Verification items for the finished model (mm, model axes). A direction names the side the tool comes from. Round coordinates to 2 decimals unless told otherwise and drop trailing zeros. Order: outer loops, then holes, each group sorted by start corner. A loop starts at its lowest first (then second) coordinate and runs counter-clockwise, first axis right, second up. Notation, with made-up numbers: M 71,31.25 L 125,31.25 A15 cw 125,57.25 Z; hole C -27.5,-5 d7. An arc over 180 degrees is marked long. One line per item, written item: value. Start each with the question number.
from build123d import *

# Parameters (mm, degrees)
F0_W        = 152.4
F0_H        = 76.2
F1_DEPTH    = 12.7
F2_R        = 6.35
F3_DEPTH    = 12.701
F4_W        = 25.4
F4_H        = 50.8
F6_W        = 11.3594501876
F6_H        = 17.78
F8_R        = 5.08
F9_T1_DEPTH = 102.3282991577
F9_T3_DEPTH = 178.5282991577


# Not quite as in the source:
# - a fillet or chamfer that OpenCascade refuses, or shapes differently, is made with other operations: its cross-section is extruded or revolved along the edge and cut away or added


with BuildPart() as f1:
    # F0 (on Top) → F1 (new body)
    with BuildSketch(Plane.XY):
        Rectangle(F0_W, F0_H)
    extrude(amount=F1_DEPTH)

    # F2 (on face) → F3 (cut, through all)
    with BuildSketch(Plane.XY.offset(12.7)):
        with Locations((-63.9521719884, 28.7373781539)):
            Circle(F2_R)
        with Locations((-65.762154874, -27.1426218461)):
            Circle(F2_R)
        with Locations((63.0478280116, 28.7373781539)):
            Circle(F2_R)
        with Locations((61.237845126, -27.1426218461)):
            Circle(F2_R)
    extrude(amount=-F3_DEPTH, mode=Mode.SUBTRACT)

    # F4 (on Front) → F5 (revolve)
    with BuildSketch(Plane.XZ):
        with Locations((12.7, 38.1)):
            Rectangle(F4_W, F4_H)
    revolve(axis=Axis((0, 0, 38.1), (0, 0, 1)))

    # F6 (on Front) → F7 (revolve, cut)
    with BuildSketch(Plane.XZ):
        with Locations((25.2974471077, 38.0985615775)):
            Rectangle(F6_W, F6_H)
    revolve(axis=Axis((0, 0, 12.7), (0, 0, 1)), mode=Mode.SUBTRACT)

    # F8
    f8_edges = [f1.edges().sort_by_distance(p)[0] for p in [
        (-25.4, 0, 63.5),
        (-25.4, 0, 12.7),
    ]]
    fillet(f8_edges, radius=F8_R)

    # F9: chamfer of 5.08 on 4 edges, made by hand

    # F9_s2 → F9_t1 (cut)
    with BuildSketch(Plane.XZ.offset(-51.1641495789)):
        Polygon((71.12, 12.7), (76.2, 7.62), (76.2, 12.7), align=None)
        Polygon((-71.12, 12.7), (-76.2, 7.62), (-76.2, 12.7), align=None)
    extrude(amount=F9_T1_DEPTH, mode=Mode.SUBTRACT)

    # F9_s4 → F9_t3 (cut)
    with BuildSketch(Plane.YZ.offset(-89.2641495789)):
        Polygon((33.02, 12.7), (38.1, 7.62), (38.1, 12.7), align=None)
        Polygon((-33.02, 12.7), (-38.1, 7.62), (-38.1, 12.7), align=None)
    extrude(amount=F9_T3_DEPTH, mode=Mode.SUBTRACT)


solid = f1.part
1. Depth check by flat-ended pin: pin 1 (4 mm diameter, centred on y = -13, z = 55, fed in from +X); pin 2 (20.5 mm diameter, centred on x = -63.95, y = 28.74, fed in from +Z); pin 3 (5 mm diameter, centred on x = -19.5, z = 35, fed in from -Y); pin 4 (12 mm diameter, centred on x = -16, y = -1, fed in from -Z). Enter the tip coordinate at first touch or a pass-through.
2. Draft check along Y on faces 1 (the face through (73.62, 0.53, 10.2)), 2 (the face through (-65.33, 22.54, 6.44)), 3 (the face through (-1.07, 35.52, 10.2)), 4 (the face through (-59.896, -29.575, 6.439)). Enter one of: released by +Y, released by -Y, zero draft, split by the parting line, or undercut.
3. Section check C-C (z = 35). Record the cut outline in (x, y).
4. Scan lines: line 1 along X through (y, z) = (25.5, 4); line 2 along X through (y, z) = (-29.5, 5.5); line 3 along Z through (x, y) = (-36.5, -24.5). Record each from-to range of solid material in increasing order.
5. Section check A-A (x = 0). Record the cut outline in (y, z), and give its area (3 significant figures).
6. Tool access check on faces 5 (the face through (-1.07, -35.52, 10.2)), 6 (the face through (-13, -15, 29.209)), 7 (the face through (-5.506, -24.796, 23.574)). Record the directions out of +Z, -Z, +X, -X, +Y, -Y that give a thin tool (end or side, any length) a straight path to the whole face; none if there is none.
7. Section check B-B (z = 6). Record the cut outline in (x, y), and give its area (3 significant figures).
8. Section check D-D (z = 53). Record the cut outline in (x, y), and give its area (3 significant figures).
Geometry check:
1. pin 1: stops at x = 22.89
1. pin 2: stops at z = 12.7
1. pin 3: stops at y = -9.79
1. pin 4: stops at z = 0
2. face 1: zero draft
2. face 2: undercut
2. face 3: released by +Y
2. face 4: undercut
3. outline: C 0,0 d39.24
4. line 1: x = -76.2 to -69.41, -58.49 to 57.59, 68.51 to 76.2
4. line 2: x = -76.2 to -71.66, -59.87 to 55.34, 67.13 to 76.2
4. line 3: z = 0 to 12.7
5. outline: M -38.1,0 L 38.1,0 L 38.1,7.62 L 33.02,12.7 L 30.48,12.7 A5.08 cw 25.4,17.78 L 25.4,29.21 L 19.62,29.21 L 19.62,46.99 L 25.4,46.99 L 25.4,58.42 A5.08 ccw 20.32,63.5 L -20.32,63.5 A5.08 ccw -25.4,58.42 L -25.4,46.99 L -19.62,46.99 L -19.62,29.21 L -25.4,29.21 L -25.4,17.78 A5.08 cw -30.48,12.7 L -33.02,12.7 L -38.1,7.62 Z
5. area: 3,320 mm²
6. face 5: +Z, +X, -X, -Y
6. face 6: none
6. face 7: +Z
7. outline: M -76.2,-38.1 L 76.2,-38.1 L 76.2,38.1 L -76.2,38.1 Z; hole C -65.76,-27.14 d12.7; hole C -63.95,28.74 d12.7; hole C 61.24,-27.14 d12.7; hole C 63.05,28.74 d12.7
7. area: 11,100 mm²
8. outline: C 0,0 d50.8
8. area: 2,030 mm²
